Source: CAD feature listing. Evaluate the final solid. Frame: model axes, mm. Coordinates: 2 decimals unless noted, no trailing zeros. Order: outer loops, then holes, each group sorted by start corner. A loop starts at its lowest first (then second) coordinate and runs counter-clockwise, first axis right, second up.
```python
from build123d import *

# Parameters (mm, degrees)
SKETCH1_R                    = 4.7625
BOSS_EXTRUDE1_DEPTH          = 4.762
SKETCH5_R                    = 1.9304
MOTOR_MOUNTING_HOLES_DEPTH   = 5.762
SKETCH7_R                    = 1.5875
ARDUINO_MOUNTING_HOLES_DEPTH = 5.762
HANDLES_DEPTH                = 5.762


with BuildPart() as part:
    # Sketch1 → Boss-Extrude1 (new body)
    with BuildSketch(Plane.XY):
        with BuildLine():
            Line((135.64320405, -94.121895407), (130.632187999, -75.420528906))
            Line((130.632187999, -75.420528906), (149.3335545, -70.409512855))
            ThreePointArc((149.3335545, -70.409512855), (-45.751779591, 158.634122005), (-88.90313596, -139.119525648))
            ThreePointArc((-88.90313596, -139.119525648), (-82.55, -142.980794165), (-76.029475394, -146.552137041))
            ThreePointArc((-76.029475394, -146.552137041), (39.694857608, -160.257069359), (135.64320405, -94.121895407))
        make_face()
        with Locations((0, -157.49999996)):
            Circle(SKETCH1_R, mode=Mode.SUBTRACT)
        with Locations((-136.399001061, 78.74999998)):
            Circle(SKETCH1_R, mode=Mode.SUBTRACT)
        with Locations((136.399001061, 78.74999998)):
            Circle(SKETCH1_R, mode=Mode.SUBTRACT)
    extrude(amount=BOSS_EXTRUDE1_DEPTH)

    # Sketch5 → motor_mounting_holes (cut, through all)
    with BuildSketch(Plane.XY.offset(4.762)):
        with Locations((-114.020939706, 65.753939357)):
            Circle(SKETCH5_R)
        with Locations((-81.776804288, 74.490196087)):
            Circle(SKETCH5_R)
        with Locations((-105.284682976, 33.50980394)):
            Circle(SKETCH5_R)
    extrude(amount=-MOTOR_MOUNTING_HOLES_DEPTH, mode=Mode.SUBTRACT)

    # Sketch7 → arduino mounting holes (cut, through all)
    with BuildSketch(Plane(origin=(0, 0, 0), x_dir=(-1, 0, 0), z_dir=(0, 0, -1))):
        with Locations((-13.114276913, -15.277418882)):
            Circle(SKETCH7_R)
        with Locations((8.521314036, -62.911361657)):
            Circle(SKETCH7_R)
        with Locations((11.082472869, -1.307418882)):
            Circle(SKETCH7_R)
        with Locations((49.680700023, -37.681509395)):
            Circle(SKETCH7_R)
    extrude(amount=-ARDUINO_MOUNTING_HOLES_DEPTH, mode=Mode.SUBTRACT)

    # Sketch8 → handles (cut, through all)
    with BuildSketch(Plane.XY.offset(4.762)):
        with BuildLine():
            Line((12.087922967, 138.165591749), (10.53352986, 120.398797227))
            ThreePointArc((10.53352986, 120.398797227), (12.604919715, 113.314590764), (18.92461727, 109.501709969))
            ThreePointArc((18.92461727, 109.501709969), (55.5625, 96.237072996), (85.368953956, 71.140054298))
            ThreePointArc((85.368953956, 71.140054298), (91.830854363, 67.573476067), (99.001652054, 69.321703063))
            Line((99.001652054, 69.321703063), (113.6109509, 79.551244243))
            ThreePointArc((113.6109509, 79.551244243), (117.84686521, 86.476490147), (115.658001653, 94.293834786))
            ThreePointArc((115.658001653, 94.293834786), (74.6125, 129.23264088), (23.831855518, 147.309684975))
            ThreePointArc((23.831855518, 147.309684975), (15.967404692, 145.296624102), (12.087922967, 138.165591749))
        make_face()
        with BuildLine():
            Line((-113.6109509, -79.551244243), (-99.001652054, -69.321703063))
            ThreePointArc((-99.001652054, -69.321703063), (-91.830854363, -67.573476067), (-85.368953956, -71.140054298))
            ThreePointArc((-85.368953956, -71.140054298), (-55.5625, -96.237072996), (-18.92461727, -109.501709969))
            ThreePointArc((-18.92461727, -109.501709969), (-12.604919715, -113.314590764), (-10.53352986, -120.398797227))
            Line((-10.53352986, -120.398797227), (-12.087922967, -138.165591749))
            ThreePointArc((-12.087922967, -138.165591749), (-15.967404692, -145.296624102), (-23.831855518, -147.309684975))
            ThreePointArc((-23.831855518, -147.309684975), (-74.6125, -129.23264088), (-115.658001653, -94.293834786))
            ThreePointArc((-115.658001653, -94.293834786), (-117.84686521, -86.476490147), (-113.6109509, -79.551244243))
        make_face()
    extrude(amount=-HANDLES_DEPTH, mode=Mode.SUBTRACT)


solid = part.part
```
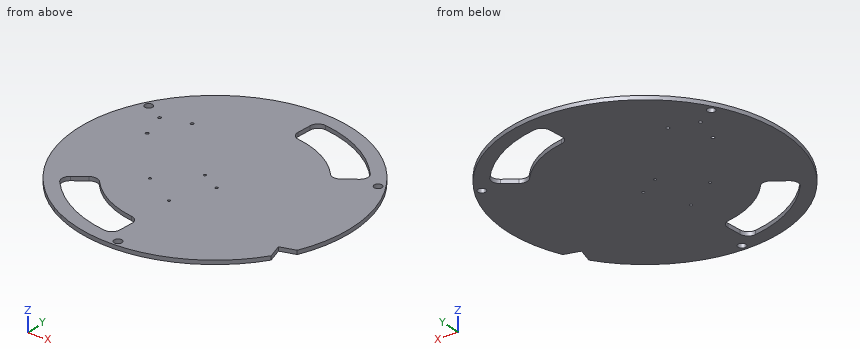
Q1. Section query B-B on z = 0.75. Give the number of separate pieces and of enclosed holes in the cut face, plus the area to 3 significant figures.
Solutions:
separate pieces: 1
enclosed holes: 12
area: 76,700 mm2
Q2. Section query A-A on x = 0. Output: boundary loops of the cut face in (y, z), plus the area to 3 significant figures.
Solutions:
outline: (-165.1, 0) - (-162.26, 0) - (-162.26, 4.76) - (-165.1, 4.76) - close; (-152.74, 0) - (165.1, 0) - (165.1, 4.76) - (-152.74, 4.76) - close
area: 1,530 mm2
Q3. Section query C-C on y = -157.5. Output: boundary loops of the cut face in (x, z).
Solutions:
outline: (-49.52, 0) - (-4.76, 0) - (-4.76, 4.76) - (-49.52, 4.76) - close; (4.76, 0) - (49.52, 0) - (49.52, 4.76) - (4.76, 4.76) - close
Q4. Section query D-D on y = 40.5. Output: boundary loops of the cut face in (x, z), plus the area to 3 significant figures.
Solutions:
outline: (-160.06, 0) - (160.06, 0) - (160.06, 4.76) - (-160.06, 4.76) - close
area: 1,520 mm2
Q5. Material intervals for line 1 along Y through (x, z) = (-49.5, 1.4); line 2 along Y through (x, z) = (18, 1.9); line 3 along Y through (x, z) = (-110, 3.55), sorted ascending.
Solutions:
line 1: y = -157.5 to -140.78, -99.49 to -39.26, -36.1 to 157.5
line 2: y = -164.12 to 109.71, 146.53 to 164.12
line 3: y = -123.12 to -100.84, -77.02 to 123.12
Q6. Pin query (flat end, axial travel): P1, Ø1.5, axis at x = -94.5, z = 1, coming from the -Y side; P2, Ø15, axis at x = -136.4, y = 78.75, coming from the -Z side; P3, Ø1.5, axis at y = 13, z = 1.5, coming from the +X side. Return the tip coordinate at first contact, or that it passes through.
Solutions:
P1: stops at y = -135.9
P2: stops at z = 0
P3: stops at x = 164.64
